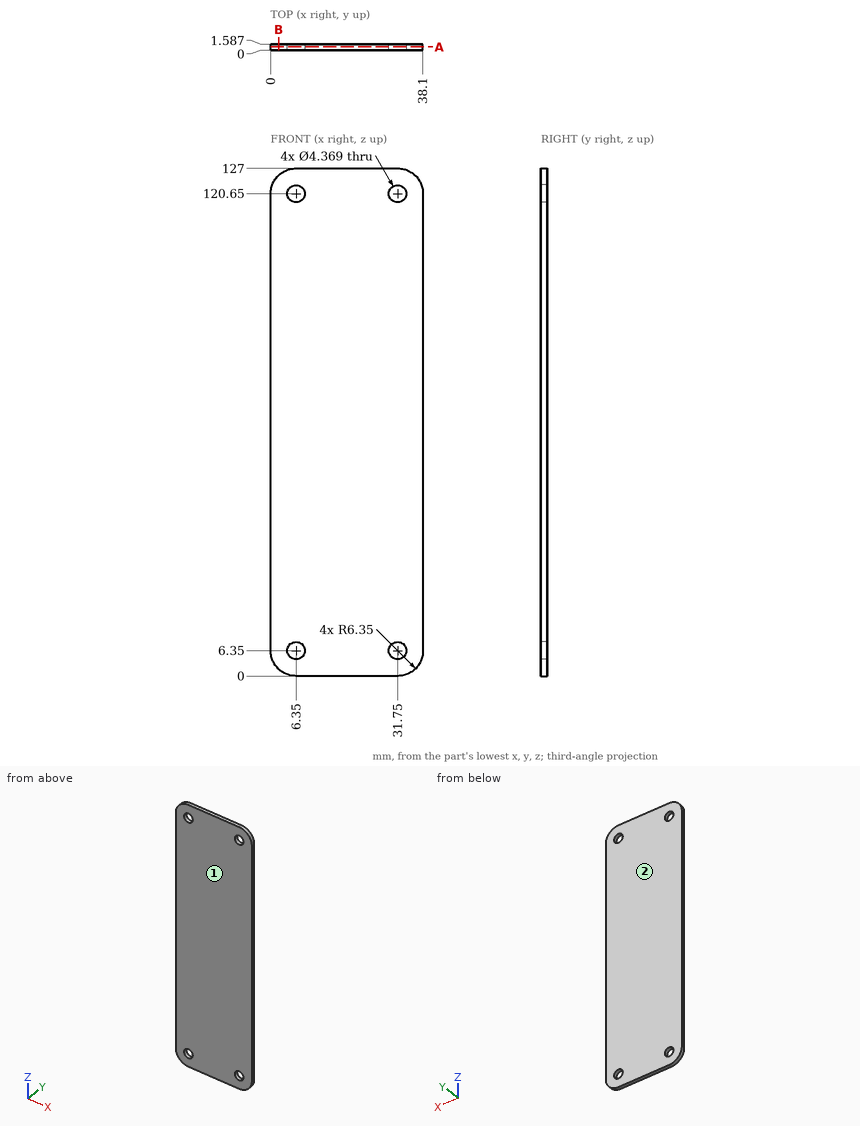
For this review, use the dimensioned drawing (mm, ordinates from the lowest corner) and the shaded views. Round coordinates to 2 decimals unless told otherwise and drop trailing zeros. Write each loop counter-clockwise with the first axis right and the second up, starting at its lowest first coordinate (ties: lowest second). Pieces come first, ordered by that corner, then holes. Notation, with made-up numbers: M 72.5,73 L 127.5,73 A31 ccw 127.5,99 Z; hole C 44,36.25 d3. An arc over 180 degrees is marked long. Write item = value, one per line. Start each with the question number.
(1) We need section A-A (y = 0.85). Give the number of separate pieces and of enclosed holes in the cut face, then the cut area to 3 significant figures.
(2) The part is to be moulded in two halves that separate along Y. For the marked faces 1 and 2, say which applies: +Y half, -Y half, draft (parallel to the pull), parting line (faces both ways), or undercut.
(3) For line 1 along Z through (x, y) = (6.35, 1.15) (1 decimal), list the stretches that pass through material, from the lowest coordinate up.
(4) We need section B-B (x = 2). Give the boundary of the cut face in (y, z), then the cut area to 3 significant figures.
Results found:
q1.separate_pieces = 1
q1.enclosed_holes = 4
q1.area = 4,740 mm²
q2.face_1 = -Y half
q2.face_2 = +Y half
q3.line_1 = 0 to 4.2, 8.5 to 118.5, 122.8 to 127
q4.outline = M 0,1.72 L 1.59,1.72 L 1.59,125.28 L 0,125.28 Z
q4.area = 196 mm²
